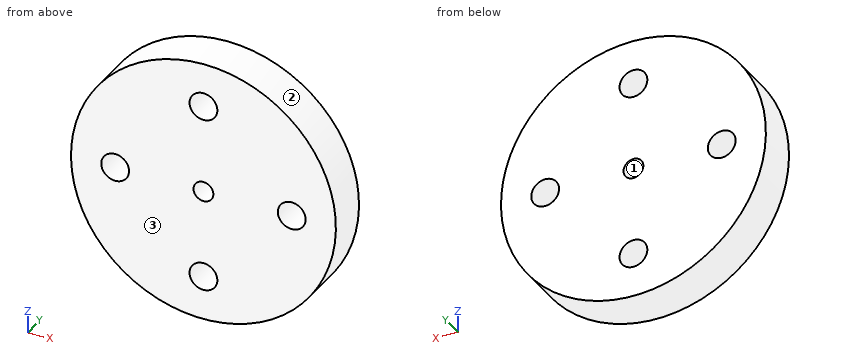
```python
from build123d import *

# Parameters (mm, degrees)
SKETCH1_R           = 30
BOSS_EXTRUDE1_DEPTH = 10
SKETCH3_R           = 3.15
CUT_EXTRUDE2_DEPTH  = 44.588989435
SKETCH4_R           = 2.25
CUT_EXTRUDE3_DEPTH  = 10


with BuildPart() as part:
    # Sketch1 → Boss-Extrude1 (new body)
    with BuildSketch(Plane(origin=(0, 0, 0), x_dir=(1, 0, 0), z_dir=(0, 1, 0))):
        with Locations(Location((0, 0, 0), (0, 0, 270))):
            Circle(SKETCH1_R)
    extrude(amount=BOSS_EXTRUDE1_DEPTH)

    # Sketch3 → Cut-Extrude2 (cut, through all)
    with BuildSketch(Plane(origin=(0, 10, 0), x_dir=(1, 0, 0), z_dir=(0, 1, 0))):
        with Locations(Location((0, 20, 0), (0, 0, 270))):
            Circle(SKETCH3_R)
        with Locations(Location((20, 0, 0), (0, 0, 270))):
            Circle(SKETCH3_R)
        with Locations(Location((0, -20, 0), (0, 0, 270))):
            Circle(SKETCH3_R)
        with Locations(Location((-20, 0, 0), (0, 0, 270))):
            Circle(SKETCH3_R)
    extrude(amount=-CUT_EXTRUDE2_DEPTH, mode=Mode.SUBTRACT)

    # Sketch4 → Cut-Extrude3 (cut)
    with BuildSketch(Plane(origin=(0, 10, 0), x_dir=(1, 0, 0), z_dir=(0, 1, 0))):
        with Locations(Location((0, 0, 0), (0, 0, 270))):
            Circle(SKETCH4_R)
    extrude(amount=-CUT_EXTRUDE3_DEPTH, mode=Mode.SUBTRACT)


solid = part.part
```
Check sheet for the modelled part. Datum: model origin and axes. Units: mm. Face numbers are marked on the shaded views. Coordinates: 2 decimals unless noted, no trailing zeros. Loops run counter-clockwise (first coordinate to the right, second up) from the corner with the lowest first, then second, coordinate; pieces in that order, holes last.
1) Gauge pin test, flat ends, axial feed: pin 1 (5 mm diameter, centred on y = 3, z = -11, fed in from -X); pin 2 (4 mm diameter, centred on x = 0, z = 20, fed in from -Y); pin 3 (1 mm diameter, centred on x = -4, y = 2, fed in from +Z); pin 4 (1.5 mm diameter, centred on y = 7.5, z = -21.5, fed in from -X). Record the tip position at first contact, or that the pin passes through.
2) Sectioned sample at A-A (z = 0). Record the boundary of the cut face in (x, y).
3) Material ranges on probe 1 along Z at (x, y) = (-1.5, 8.25); probe 2 along Z at (x, y) = (-0.5, 4.25); probe 3 along X at (y, z) = (1, 20), recorded low to high.
4) Sectioned sample at B-B (x = 0). Record the boundary of the cut face in (y, z), and give its area (3 significant figures).
5) Sectioned sample at D-D (y = 6). Record the boundary of the cut face in (x, z).
6) Release check for a two-part mould opening along X. For the marked faces 1, 2 and 3 record: released by +X, released by -X, zero draft, split by the parting line, or undercut.
7) Sectioned sample at C-C (x = 20). Record the boundary of the cut face in (y, z).
Check sheet entries:
1. pin 1: stops at x = -28.77
1. pin 2: passes through
1. pin 3: stops at z = 29.8
1. pin 4: stops at x = -21.67
2. outline: (-30, 0) - (-23.15, 0) - (-23.15, 10) - (-30, 10) - close; (-16.85, 0) - (-2.25, 0) - (-2.25, 10) - (-16.85, 10) - close; (2.25, 0) - (16.85, 0) - (16.85, 10) - (2.25, 10) - close; (23.15, 0) - (30, 0) - (30, 10) - (23.15, 10) - close
3. probe 1: z = -29.96 to -22.77, -17.23 to -1.68, 1.68 to 17.23, 22.77 to 29.96
3. probe 2: z = -30 to -23.11, -16.89 to -2.19, 2.19 to 16.89, 23.11 to 30
3. probe 3: x = -22.36 to -3.15, 3.15 to 22.36
4. outline: (0, -30) - (10, -30) - (10, -23.15) - (0, -23.15) - close; (0, -16.85) - (10, -16.85) - (10, -2.25) - (0, -2.25) - close; (0, 2.25) - (10, 2.25) - (10, 16.85) - (0, 16.85) - close; (0, 23.15) - (10, 23.15) - (10, 30) - (0, 30) - close
4. area: 429 mm2
5. outline: circle Ø60 at (0, 0); hole circle Ø6.3 at (-20, 0); hole circle Ø6.3 at (0, -20); hole circle Ø6.3 at (0, 20); hole circle Ø4.5 at (0, 0); hole circle Ø6.3 at (20, 0)
6. face 1: undercut
6. face 2: split by the parting line
6. face 3: zero draft
7. outline: (0, -22.36) - (10, -22.36) - (10, -3.15) - (0, -3.15) - close; (0, 3.15) - (10, 3.15) - (10, 22.36) - (0, 22.36) - close
